Geometry check sheet. Reference: the model listing, model coordinates, mm. Face numbers are marked on the shaded views. A direction names the side the tool comes from. Round coordinates to 2 decimals unless told otherwise and drop trailing zeros. Write each loop counter-clockwise with the first axis right and the second up, starting at its lowest first coordinate (ties: lowest second). Pieces come first, ordered by that corner, then holes. Notation, with made-up numbers: (70.25, -12) -> (83.25, -12) arc R19 ccw to (83.25, 11) -> close; hole circle Ø8 at (67, 32.5). An arc over 180 degrees is marked (long way). Use a Markdown table: item, result.
```python
from build123d import *

# Parameters (mm, degrees)
SKETCH1_R           = 8.5
SKETCH1_R_2         = 2
BOSS_EXTRUDE1_DEPTH = 5
SKETCH2_R           = 8.5
SKETCH2_R_2         = 5
BOSS_EXTRUDE2_DEPTH = 20
SKETCH3_R           = 2
BOSS_EXTRUDE3_DEPTH = 3
CHAMFER1_SIZE       = 1
CUT_EXTRUDE1_REACH  = 19
SKETCH4_R           = 2


with BuildPart() as part:
    # Sketch1 → Boss-Extrude1 (new body)
    with BuildSketch(Plane.XY):
        Circle(SKETCH1_R)
        Circle(SKETCH1_R_2, mode=Mode.SUBTRACT)
    extrude(amount=BOSS_EXTRUDE1_DEPTH)

    # Sketch2 → Boss-Extrude2 (add)
    with BuildSketch(Plane.XY.offset(5)):
        Circle(SKETCH2_R)
        Circle(SKETCH2_R_2, mode=Mode.SUBTRACT)
    extrude(amount=BOSS_EXTRUDE2_DEPTH)

    # Sketch3 → Boss-Extrude3 (add)
    with BuildSketch(Plane(origin=(0, 0, 0), x_dir=(-1, 0, 0), z_dir=(0, 0, -1))):
        Polygon((-4.500595024, 1.03825708), (-3.149454519, -3.378501083), (1.351140505, -4.416758163), (4.500595024, -1.03825708), (3.149454519, 3.378501083), (-1.351140505, 4.416758163), align=None)
        Circle(SKETCH3_R, mode=Mode.SUBTRACT)
    extrude(amount=BOSS_EXTRUDE3_DEPTH)

    # Chamfer1
    chamfer1_edges = [part.edges().sort_by_distance(p)[0] for p in [
        (-8.5, 0, 25),
    ]]
    chamfer(chamfer1_edges, length=CHAMFER1_SIZE)

    # Sketch4 → Cut-Extrude1 (cut, up to next)
    with BuildSketch(Plane(origin=(8.5, 0, 0), x_dir=(0, 0, -1), z_dir=(1, 0, 0)), mode=Mode.PRIVATE) as cut_extrude1_sk1:
        with Locations((-18, 0)):
            Circle(SKETCH4_R)
    cut_extrude1_tool1 = extrude(cut_extrude1_sk1.sketch, amount=-CUT_EXTRUDE1_REACH, mode=Mode.PRIVATE) & part.part
    add(cut_extrude1_tool1.solids().sort_by_distance((8.5, 0, 18))[0], mode=Mode.SUBTRACT)


solid = part.part
```
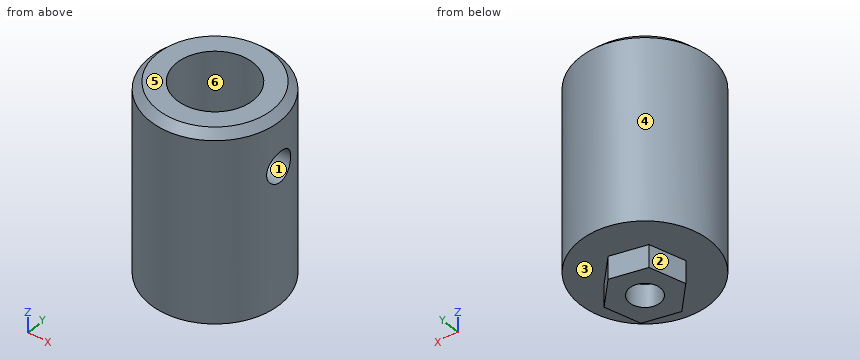
(1) Release check for a two-part mould opening along Y. For the marked faces 4, 5 and 6 record: +Y half, -Y half, draft (parallel to the pull), parting line (faces both ways), or undercut.
A:
| item | result |
|---|---|
| face 4 | parting line |
| face 5 | draft |
| face 6 | undercut |
(2) Section check D-D on z = 18. Record the cut outline in (x, y), plus the area to 3 significant figures.
A:
| item | result |
|---|---|
| outline | (4.58, -2) arc R5 cw (long way) to (4.58, 2) -> (8.26, 2) arc R8.5 ccw (long way) to (8.26, -2) -> close |
| area | 134 mm2 |
(3) Section check C-C on x = 0. Record the cut outline in (y, z).
A:
| item | result |
|---|---|
| outline | (-8.5, 0) -> (-4.11, 0) -> (-4.11, -3) -> (-2, -3) -> (-2, 5) -> (-5, 5) -> (-5, 25) -> (-7.5, 25) -> (-8.5, 24) -> close; (2, -3) -> (4.11, -3) -> (4.11, 0) -> (8.5, 0) -> (8.5, 24) -> (7.5, 25) -> (5, 25) -> (5, 5) -> (2, 5) -> close |
(4) Gauge pin test, flat ends, axial feed: pin 1 Ø4 at (y, z) = (-5.5, 19) entering from -X; pin 2 Ø5 at (x, y) = (-1.5, -0.5) entering from +Z; pin 3 Ø1 at (y, z) = (1, 11.5) entering from -X. Record the tip position at first contact, or that the pin passes through.
A:
| item | result |
|---|---|
| pin 1 | stops at x = -7.75 |
| pin 2 | stops at z = 5 |
| pin 3 | stops at x = -8.49 |
(5) Section check B-B on z = 1.25. Record the cut outline in (x, y).
A:
| item | result |
|---|---|
| outline | circle Ø17 at (0, 0); hole circle Ø4 at (0, 0) |
(6) Section check A-A on y = 0. Record the cut outline in (x, z).
A:
| item | result |
|---|---|
| outline | (-8.5, 0) -> (-4.18, 0) -> (-4.18, -3) -> (-2, -3) -> (-2, 5) -> (-5, 5) -> (-5, 25) -> (-7.5, 25) -> (-8.5, 24) -> close; (2, -3) -> (4.18, -3) -> (4.18, 0) -> (8.5, 0) -> (8.5, 16) -> (5, 16) -> (5, 5) -> (2, 5) -> close; (5, 20) -> (8.5, 20) -> (8.5, 24) -> (7.5, 25) -> (5, 25) -> close |
(7) Thickness scan on line 1 (Y direction, x = 0.25, z = 18.25); line 2 (Z direction, x = 2.5, y = 2.5); line 3 (Y direction, x = 2, z = 23.5). Record the ranges inside material, lowest first.
A:
| item | result |
|---|---|
| line 1 | y = -8.5 to -4.99, 4.99 to 8.5 |
| line 2 | z = -3 to 5 |
| line 3 | y = -8.26 to -4.58, 4.58 to 8.26 |
(8) Access from +Z, -Z, +X, -X, +Y, -Y to the whole of each face (thin tool, end or side, straight path). Record for the marked faces 1, 2 and 3.
A:
| item | result |
|---|---|
| face 1 | +X |
| face 2 | -Z, -X, +Y |
| face 3 | -Z |
